Print and shaded views of the part. All mm, measured from the part's lowest x, y and z. A direction names the side the tool comes from. Give positions to 0.01 mm unless a question says otherwise; leave off trailing zeros. Write each loop counter-clockwise with the first axis right and the second up, starting at its lowest first coordinate (ties: lowest second). Pieces come first, ordered by that corner, then holes. Notation, with made-up numbers: (19, -13) -> (42, -13) arc R26 ccw to (42, 15) -> close; hole circle Ø9 at (-11.5, -32). An arc over 180 degrees is marked (long way). Put each result on its own line as item: value.
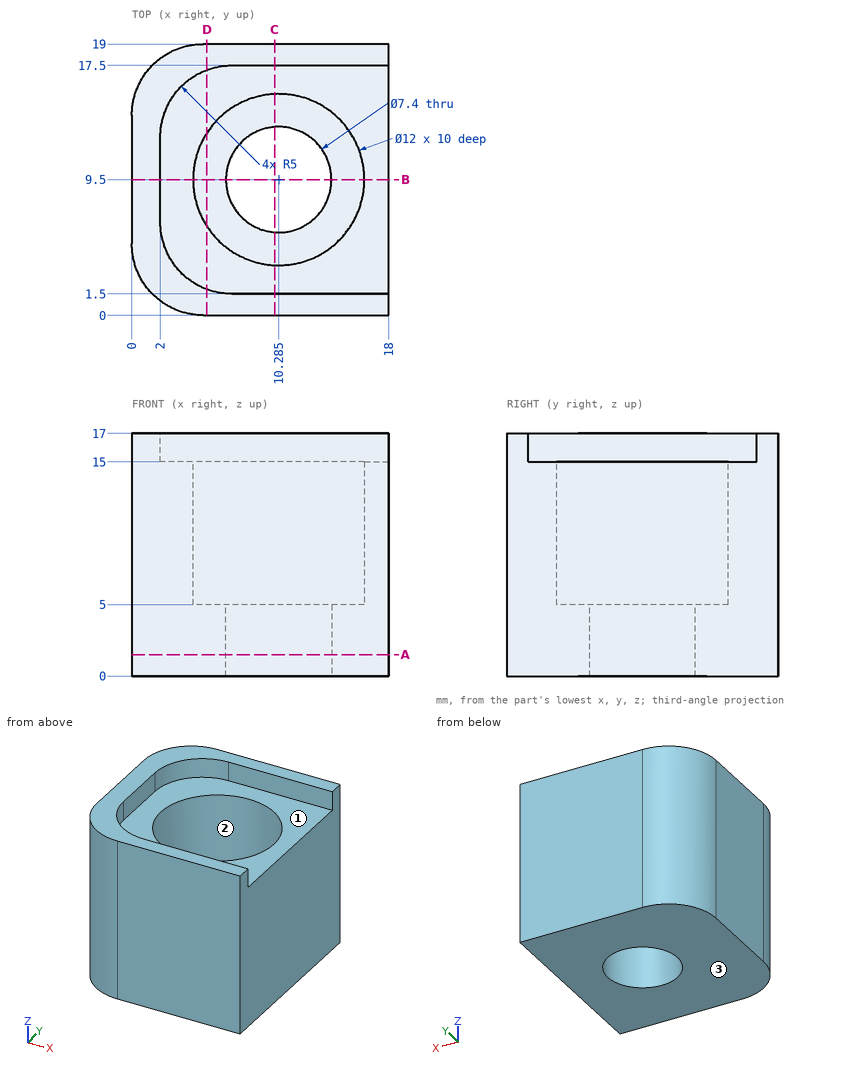
1) Pin check, flat tips, straight feed: pin 1 (8 mm diameter, centred on x = 11.5, y = 7.5, fed in from +Z); pin 2 (0.6 mm diameter, centred on y = 8.5, z = 16, fed in from +X). Stop position of each tip, or through.
Filled sheet:
pin 1: z = 15
pin 2: x = 2
2) Slice it at C-C (x = 10). Write the cut outline in (y, z), plus the area to 3 significant figures.
Filled sheet:
outline: (0, 0) -> (5.81, 0) -> (5.81, 5) -> (3.51, 5) -> (3.51, 15) -> (1.5, 15) -> (1.5, 17) -> (0, 17) -> close; (13.19, 0) -> (19, 0) -> (19, 17) -> (17.5, 17) -> (17.5, 15) -> (15.49, 15) -> (15.49, 5) -> (13.19, 5) -> close
area: 134 mm2
3) Slice it at B-B (y = 9.5). Write the cut outline in (x, z) (3 decimals), plus the area to 3 significant figures.
Filled sheet:
outline: (0, 0) -> (6.585, 0) -> (6.585, 5) -> (4.285, 5) -> (4.285, 15) -> (2, 15) -> (2, 17) -> (0, 17) -> close; (13.985, 0) -> (18, 0) -> (18, 15) -> (16.285, 15) -> (16.285, 5) -> (13.985, 5) -> close
area: 117 mm2
4) Wall check: L1, parallel to X at y = 9.75, z = 5.5; L2, parallel to Y at x = 7, z = 16; L3, parallel to Y at x = 8.5, z = 9. Give the ranges that are in metal, low to high.
Filled sheet:
L1: 0 to 4.29, 16.28 to 18
L2: 0 to 1.5, 17.5 to 19
L3: 0 to 3.77, 15.23 to 19
5) Tool access for the marked faces 1, 2 and 3: list every direction of +Z, -Z, +X, -X, +Y, -Y with a clear straight run to the whole face (end or side of a thin tool).
Filled sheet:
face 1: +Z, +X
face 2: +Z
face 3: -Z, +X, -X, +Y, -Y
6) Slice it at A-A (z = 1.5). Write the cut outline in (x, y) (3 decimals), plus the area to 3 significant figures.
Filled sheet:
outline: (0, 5) arc R5 ccw to (5, 0) -> (18, 0) -> (18, 19) -> (5, 19) arc R5 ccw to (0, 14) -> close; hole circle Ø7.4 at (10.285, 9.5)
area: 288 mm2
7) Slice it at D-D (x = 5.25). Write the cut outline in (y, z).
Filled sheet:
outline: (0, 0) -> (19, 0) -> (19, 17) -> (17.18, 17) -> (17.18, 15) -> (12.76, 15) -> (12.76, 5) -> (6.24, 5) -> (6.24, 15) -> (1.82, 15) -> (1.82, 17) -> (0, 17) -> close
